Could you check a few things on this model? Use its own coordinates, in mm. Face numbers are marked on the shaded views. Give positions to 0.01 mm unless a question says otherwise; leave off trailing zeros. Loops run counter-clockwise (first coordinate to the right, second up) from the corner with the lowest first, then second, coordinate; pieces in that order, holes last. Notation, with made-up numbers: (26.25, -28.5) -> (71.25, -28.5) arc R34 cw to (71.25, 1.5) -> close; hole circle Ø2 at (26, 60.5). An arc over 180 degrees is marked (long way). Put each result on its own line as item: value.
```python
from build123d import *

# Parameters (mm, degrees)
PAD001_DEPTH      = 390
SKETCH003_R       = 4
HOLE_DEPTH        = 25
HOLE_TIPS_R       = 4
SKETCH004_R       = 4
HOLE001_DEPTH     = 25
HOLE001_TIPS_R    = 4
POCKET_DEPTH      = 64
POCKET_DEPTH_BACK = 5


with BuildPart() as part:
    # Sketch002 → Pad001 (new body)
    with BuildSketch(Plane.XZ):
        with BuildLine():
            ThreePointArc((25, -12.5), (28.535534, -11.035534), (30, -7.5))
            Line((30, 7.5), (30, -7.5))
            ThreePointArc((30, 7.5), (28.535534, 11.035534), (25, 12.5))
            Line((-25, 12.5), (25, 12.5))
            ThreePointArc((-25, 12.5), (-28.535534, 11.035534), (-30, 7.5))
            Line((-30, -7.5), (-30, 7.5))
            ThreePointArc((-30, -7.5), (-28.535534, -11.035534), (-25, -12.5))
            Line((25, -12.5), (-25, -12.5))
        make_face()
    extrude(amount=-PAD001_DEPTH)

    # Sketch003 (on Face9 of Pad001) → Hole (cut)
    with BuildSketch(Plane.XZ):
        with Locations((15, 0)):
            Circle(SKETCH003_R)
        with Locations((-15, 0)):
            Circle(SKETCH003_R)
    extrude(amount=-HOLE_DEPTH, mode=Mode.SUBTRACT)

    # Hole tips → Hole tip 1 section 0
    with BuildSketch(Plane.XZ.offset(-25), mode=Mode.PRIVATE) as hole_tip_1_s0:
        with Locations((15, 0)):
            Circle(HOLE_TIPS_R)
    loft([hole_tip_1_s0.sketch, Vertex(15, 27.403442, 0)], mode=Mode.SUBTRACT)

    # Hole tips → Hole tip 2 section 0
    with BuildSketch(Plane.XZ.offset(-25), mode=Mode.PRIVATE) as hole_tip_2_s0:
        with Locations((-15, 0)):
            Circle(HOLE_TIPS_R)
    loft([hole_tip_2_s0.sketch, Vertex(-15, 27.403442, 0)], mode=Mode.SUBTRACT)

    # Sketch004 (on Face5 of Hole) → Hole001 (cut)
    with BuildSketch(Plane(origin=(0, 390, 0), x_dir=(1, 0, 0), z_dir=(0, 1, 0))):
        with Locations((-15, 0)):
            Circle(SKETCH004_R)
        with Locations((15, 0)):
            Circle(SKETCH004_R)
    extrude(amount=-HOLE001_DEPTH, mode=Mode.SUBTRACT)

    # Hole001 tips → Hole001 tip 1 section 0
    with BuildSketch(Plane(origin=(0, 365, 0), x_dir=(1, 0, 0), z_dir=(0, 1, 0)), mode=Mode.PRIVATE) as hole001_tip_1_s0:
        with Locations((-15, 0)):
            Circle(HOLE001_TIPS_R)
    loft([hole001_tip_1_s0.sketch, Vertex(-15, 362.596558, 0)], mode=Mode.SUBTRACT)

    # Hole001 tips → Hole001 tip 2 section 0
    with BuildSketch(Plane(origin=(0, 365, 0), x_dir=(1, 0, 0), z_dir=(0, 1, 0)), mode=Mode.PRIVATE) as hole001_tip_2_s0:
        with Locations((15, 0)):
            Circle(HOLE001_TIPS_R)
    loft([hole001_tip_2_s0.sketch, Vertex(15, 362.596558, 0)], mode=Mode.SUBTRACT)

    # Sketch005 (on Face3 of Hole001) → Pocket (cut, two sides)
    with BuildSketch(Plane(origin=(30, 0, 0), x_dir=(0, 0, 1), z_dir=(1, 0, 0))) as pocket_sk:
        with BuildLine():
            ThreePointArc((12.5, -20), (7.5, -195), (12.5, -370))
            Line((12.5, -20), (12.5, -370))
        make_face()
    extrude(amount=-POCKET_DEPTH, mode=Mode.SUBTRACT)
    extrude(pocket_sk.sketch, amount=POCKET_DEPTH_BACK, mode=Mode.SUBTRACT)


solid = part.part
```
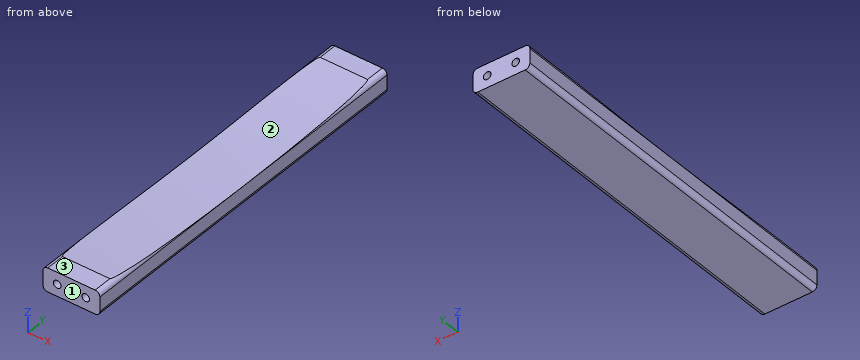
1. If we section it at C-C (y = 292): List the corners of the cut face in (x, z) for me, then the cut area to 3 significant figures.
Recorded:
outline: (-30, -7.5) arc R5 ccw to (-25, -12.5) -> (25, -12.5) arc R5 ccw to (30, -7.5) -> (30, 7.5) arc R5 ccw to (29.76, 9.04) -> (-29.76, 9.04) arc R5 ccw to (-30, 7.5) -> close
area: 1,280 mm^2
2. Thinking about a two-plate mould opening in Y: for the marked faces 1, 2 and 3, which applies, pulls with the +Y half, pulls with the -Y half, needs draft (parallel to the pull), parting line crosses it, or undercut?
Recorded:
face 1: pulls with the -Y half
face 2: undercut
face 3: needs draft
3. I need wall thicknesses on line 1 (X direction, y = 382.5, z = 0); line 2 (Z direction, x = 15, y = 19.5); line 3 (Z direction, x = 0, y = 181.5). Which ranges of each line are inside material? Lowest first, please.
Recorded:
line 1: x = -30 to -19, -11 to 11, 19 to 30
line 2: z = -12.5 to -4, 4 to 12.5
line 3: z = -12.5 to 7.53
4. I'm going to push flat-ended pins straight in: pin 1 (7 mm diameter, centred on x = -15, z = 0, fed in from -Y); pin 2 (4 mm diameter, centred on x = 14, y = 315, fed in from +Z); pin 3 (6.5 mm diameter, centred on x = 15, z = 0, fed in from -Y). Where does each tip first touch, or does it pass through?
Recorded:
pin 1: stops at y = 25.3
pin 2: stops at z = 9.93
pin 3: stops at y = 25.45
5. If we section it at A-A (x = -5.5): List the corners of the cut face in (y, z) for me, then the cut area to 3 significant figures.
Recorded:
outline: (0, -12.5) -> (390, -12.5) -> (390, 12.5) -> (370, 12.5) arc R3065 cw to (20, 12.5) -> (0, 12.5) -> close
area: 8,580 mm^2
6. If we section it at B-B (y = 241.5): List the corners of the cut face in (x, z) for me, then the cut area to 3 significant figures.
Recorded:
outline: (-30, -7.5) arc R5 ccw to (-25, -12.5) -> (25, -12.5) arc R5 ccw to (30, -7.5) -> (30, 7.5) arc R5 ccw to (29.99, 7.85) -> (-29.99, 7.85) arc R5 ccw to (-30, 7.5) -> close
area: 1,210 mm^2
